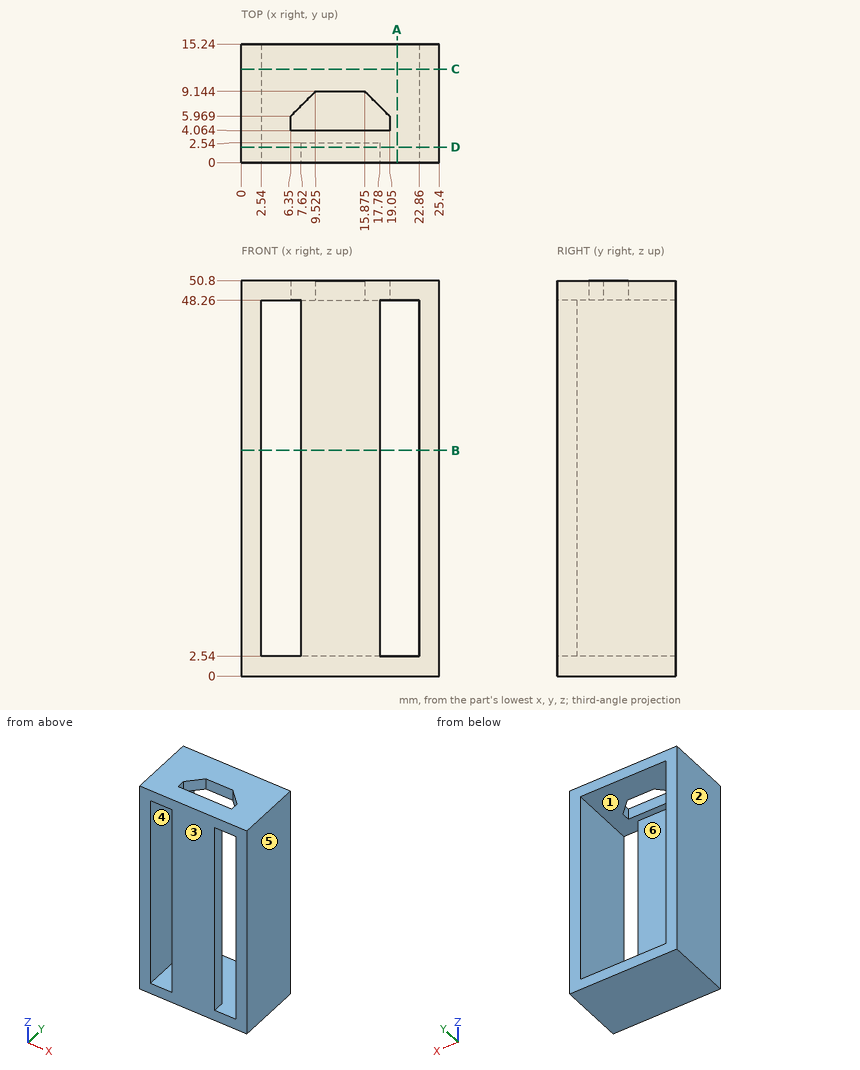
Can you work these out from the drawing? Everything is in mm from the part's minimum corner. A direction names the side the tool comes from. Coordinates: 2 decimals unless noted, no trailing zeros. Order: outer loops, then holes, each group sorted by start corner. A loop starts at its lowest first (then second) coordinate and runs counter-clockwise, first axis right, second up. Notation, with made-up numbers: (38.5, -36) -> (48.5, -36) arc R8 cw to (48.5, -28) -> close; hole circle Ø11 at (-14, 48). An arc over 180 degrees is marked (long way). Use one line per item in the form item = value.
Q1. Imagine slicing it at D-D, the plane y = 2. List the corners of the cut face in (x, z) for me.
From the geometry:
outline = (0, 0) -> (25.4, 0) -> (25.4, 50.8) -> (0, 50.8) -> close; hole (2.54, 2.54) -> (7.62, 2.54) -> (7.62, 48.26) -> (2.54, 48.26) -> close; hole (17.78, 2.54) -> (22.86, 2.54) -> (22.86, 48.26) -> (17.78, 48.26) -> close
Q2. We'd pull the mould along X, two halves only. Please class the marked faces 1, 2 and 3: released by +X, released by -X, zero draft, split by the parting line, or undercut.
From the geometry:
face_1 = undercut
face_2 = released by -X
face_3 = zero draft
Q3. Will this pin go through, and if not, where does the flat tip stop? P1, Ø11, axis at x = 13.5, z = 26, coming from the +Y side.
From the geometry:
P1 = 2.54
Q4. Imagine slicing it at A-A, the plane x = 20. List the corners of the cut face in (y, z) for me, then the cut area to 3 significant figures.
From the geometry:
outline = (0, 0) -> (15.24, 0) -> (15.24, 2.54) -> (0, 2.54) -> close; (0, 48.26) -> (15.24, 48.26) -> (15.24, 50.8) -> (0, 50.8) -> close
area = 77.4 mm²
Q5. I need wall thicknesses on L1, parallel to Z at x = 4.5, y = 12.25; L2, parallel to X at y = 13.25, z = 8; L3, parallel to Z at x = 18.75, y = 6. Which ranges of each line are inside material? Lowest first, please.
From the geometry:
L1 = 0 to 2.54, 48.26 to 50.8
L2 = 0 to 2.54, 22.86 to 25.4
L3 = 0 to 2.54
Q6. Imagine slicing it at B-B, the plane z = 29. List the corners of the cut face in (x, y) for me.
From the geometry:
outline = (0, 0) -> (2.54, 0) -> (2.54, 15.24) -> (0, 15.24) -> close; (7.62, 0) -> (17.78, 0) -> (17.78, 2.54) -> (7.62, 2.54) -> close; (22.86, 0) -> (25.4, 0) -> (25.4, 15.24) -> (22.86, 15.24) -> close
Q7. Imagine slicing it at C-C, the plane y = 12. List the corners of the cut face in (x, z) for me, then the cut area to 3 significant figures.
From the geometry:
outline = (0, 0) -> (25.4, 0) -> (25.4, 50.8) -> (0, 50.8) -> close; hole (2.54, 2.54) -> (22.86, 2.54) -> (22.86, 48.26) -> (2.54, 48.26) -> close
area = 361 mm²
Q8. Which directions (+Z, -Z, +X, -X, +Y, -Y) give clear straight access to the entire face, cutting with the end or side of a thin tool? Please do the marked faces 4, 5 and 6.
From the geometry:
face_4 = +Y, -Y
face_5 = +Z, -Z, +X, +Y, -Y
face_6 = +Y
